from build123d import *

# Parameters (mm, degrees)
F2_DEPTH = 25.4
F3_W     = 1016
F3_H     = 147.955
F4_DEPTH = 147.955
F5_DEPTH = 133.5532
F6_R     = 72.39
F7_R     = 72.39


# Not quite as in the source:
# - a feature names something its author has since deleted; it is built from what else it names


with BuildPart() as f2:
    # F1 (on face) → F2 (new body)
    with BuildSketch(Plane.XY):
        Polygon((319.0343479268, 457.2), (236.3300025423, 362.0783686638), (240.3907269744, -362.0321180929), (325.0280779844, -457.2), (1501.5633212704, -457.2), (1590.3160302528, -346.8912047778), (1588.7331709988, -205.7675014721), (1587.5366926193, 7.5891437009), (1586.3402142398, 220.9457888739), (1586.3402142398, 362.0783686638), (1508.033296253, 457.2), align=None)
        Polygon((376.3225418129, 523.0894817851), (319.0343479268, 457.2), (1508.033296253, 457.2), (1453.79114151, 523.0894817851), align=None)
        Polygon((1501.5633212704, -457.2), (325.0280779844, -457.2), (382.1802665493, -521.4630312406), (1459.5810992365, -509.3787828947), align=None)
    extrude(amount=F2_DEPTH)

    # F3 (on face) → F4 (join)
    with BuildSketch(Plane.XY.offset(25.4)):
        with Locations((895.4748051167, 428.2288251305)):
            Rectangle(F3_W, F3_H)
        with BuildLine():
            Line((1403.4748051167, 502.2063251305), (1403.4748051167, 354.2513251305))
            ThreePointArc((1403.4748051167, 354.2513251305), (1477.4523051167, 428.2288251305), (1403.4748051167, 502.2063251305))
        make_face()
        Polygon((391.4505850052, -352.5514191944), (393.1150321411, -500.4970566453), (1409.0507399579, -489.0673767425), (1407.3862928221, -341.1217392917), align=None)
        with BuildLine():
            Line((1407.3862928221, -341.1217392917), (1409.0507399579, -489.0673767425))
            ThreePointArc((1409.0507399579, -489.0673767425), (1482.1913351154, -414.2623344491), (1407.3862928221, -341.1217392917))
        make_face()
    extrude(amount=F4_DEPTH)

    # F3 (on face) → F5 (join)
    with BuildSketch(Plane.XY.offset(25.4)):
        with Locations((895.4748051167, 428.2288251305)):
            Rectangle(F3_W, F3_H)
        with BuildLine():
            Line((1403.4748051167, 502.2063251305), (1403.4748051167, 354.2513251305))
            ThreePointArc((1403.4748051167, 354.2513251305), (1477.4523051167, 428.2288251305), (1403.4748051167, 502.2063251305))
        make_face()
        Polygon((391.4505850052, -352.5514191944), (393.1150321411, -500.4970566453), (1409.0507399579, -489.0673767425), (1407.3862928221, -341.1217392917), align=None)
        with BuildLine():
            Line((1407.3862928221, -341.1217392917), (1409.0507399579, -489.0673767425))
            ThreePointArc((1409.0507399579, -489.0673767425), (1482.1913351154, -414.2623344491), (1407.3862928221, -341.1217392917))
        make_face()
    extrude(amount=F5_DEPTH)

    # F6
    f6_edges = [f2.edges().sort_by_distance(p)[0] for p in [
        (895.474805, 502.206325, 173.355),
        (1477.452305, 428.228825, 173.355),
        (895.474805, 354.251325, 173.355),
    ]]
    fillet(f6_edges, radius=F6_R)

    # F7
    f7_edges = [f2.edges().sort_by_distance(p)[0] for p in [
        (899.418439, -346.836579, 173.355),
        (1482.191335, -414.262334, 173.355),
        (901.082886, -494.782217, 173.355),
    ]]
    fillet(f7_edges, radius=F7_R)


solid = f2.part
Design review of the part built by this model. Coordinates are the model's own, in mm. A direction names the side the tool comes from. Coordinates: 2 decimals unless noted, no trailing zeros. Order: outer loops, then holes, each group sorted by start corner. A loop starts at its lowest first (then second) coordinate and runs counter-clockwise, first axis right, second up.
Item 1: Take a section at A-A, the plane z = 68. Write out the cut boundary in (x, y) (1 decimal).
Item 2: The part is to be moulded in two halves that separate along Y. For faces 4 (the cylindrical face through (892.54, -367.56, 151.59)), 5 (the flat face through (387.475, 427, 98)), 6 (the cylindrical face through (907.96, -474.06, 151.59)), 7 (the flat face through (1520.99, 441.46, 12.52)), say which applies: pulls with the +Y half, pulls with the -Y half, needs draft (parallel to the pull), parting line crosses it, or undercut.
Item 3: For line 1 (Y direction, x = 411, z = 67); line 2 (Z direction, x = 450, y = 116); line 3 (Y direction, x = 1026.5, z = 45), list the stretches that pass through material, from the lowest coordinate up.
Item 4: Take a section at B-B, the plane y = -103.5. Write out the cut boundary in (x, z).
Item 5: For pin 1 Ø6 at (y, z) = (-121, 21) entering from +X; pin 2 Ø1 at (x, z) = (1272.5, 111.5) entering from -Y; pin 3 Ø20.5 at (y, z) = (320, 11.5) entering from +X, all flat-tipped, find the tip position at first contact; note any pin that passes through.
Item 6: Take a section at C-C, the plane x = 329. Write out the cut boundary in (y, z), then the cut area to 3 significant figures.
Item 7: For faces 1 (the flat face through (888, 502.206, 63)), 2 (the flat face through (888, 354.251, 63)), 3 (the cylindrical face through (1477.434, 426.602, 62.654)), list the 3-axis set-ups (+Z, -Z, +X, -X, +Y, -Y) from which the entire face can be reached by the end or side of a thin tool; tool diameter is ignored.
The answers:
1. outline: (387.5, 354.3) - (1403.5, 354.3) arc R74 ccw to (1403.5, 502.2) - (387.5, 502.2) - close; (391.5, -352.6) - (393.1, -500.5) - (1409.1, -489.1) arc R74 ccw to (1407.4, -341.1) - close
2. face 4: undercut
2. face 5: needs draft
2. face 6: pulls with the -Y half
2. face 7: pulls with the +Y half
3. line 1: y = -500.3 to -352.33, 354.25 to 502.21
3. line 2: z = 0 to 25.4
3. line 3: y = -493.37 to -345.41, 354.25 to 502.21
4. outline: (238.94, 0) - (1588.16, 0) - (1588.16, 25.4) - (238.94, 25.4) - close
5. pin 1: stops at x = 1588.27
5. pin 2: stops at y = -489.9
5. pin 3: stops at x = 1586.34
6. outline: (-461.67, 0) - (468.66, 0) - (468.66, 25.4) - (-461.67, 25.4) - close
6. area: 23,600 mm2
7. face 1: +Z, +X, -X, +Y
7. face 2: +Z, +X, -X
7. face 3: +Z, +X
